For this review, take the finished solid that the model builds, in its own axes (mm). Face numbers are marked on the shaded views. A direction names the side the tool comes from. Give positions to 0.01 mm unless a question says otherwise; leave off trailing zeros. Order: outer loops, then holes, each group sorted by start corner. A loop starts at its lowest first (then second) coordinate and runs counter-clockwise, first axis right, second up.
Item 1: Machinability: for the marked faces 4, 5 and 6, which of the approach directions +Z, -Z, +X, -X, +Y, -Y give a long, thin tool a straight path to every point of the face, cutting with its end or side? Answer none if there is none.
Item 2: Consider section C-C (z = 0). Give the boundary of the cut face in (x, y).
Item 3: For probe 1 along Y at (x, z) = (-5.15, 0); probe 2 along Z at (x, y) = (-5.5, 13); probe 3 along Y at (x, z) = (-5.25, -0.5), list the stretches that pass through material, from the lowest coordinate up.
Item 4: Consider section A-A (x = -9). Give the boundary of the cut face in (y, z), plus the area to 3 significant figures.
Item 5: Consider section B-B (y = 10). Give the boundary of the cut face in (x, z), plus the area to 3 significant figures.
Item 6: The part is to be moulded in two halves that separate along Y. For the marked faces 1, 2 and 3, say which applies: released by +Y, released by -Y, zero draft, split by the parting line, or undercut.
Item 7: For P1, Ø1, axis at y = 9, z = 0.5, coming from the -X side; P2, Ø3, axis at y = 8.5, z = 4.5, coming from the -X side; P3, Ø1.5, axis at x = -3, y = 13, coming from the -Z side; P4, Ø2.5, axis at x = -8, y = 10, coming from the -Z side, all flat-tipped, find the tip position at first contact; note any pin that passes through.
Item 8: Consider section D-D (y = 15.25). Give the boundary of the cut face in (x, z).
```python
from build123d import *

# Parameters (mm, degrees)
BOSS_EXTRUDE1_DEPTH = 20
SKETCH2_R           = 2.1
CUT_EXTRUDE1_DEPTH  = 6


with BuildPart() as part:
    # Sketch1 → Boss-Extrude1 (new body)
    with BuildSketch(Plane(origin=(0, 0, 0), x_dir=(1, 0, 0), z_dir=(0, 1, 0))):
        with BuildLine():
            Line((-4.847127702, 5.487127702), (-4.847127702, 2.63))
            Line((-4.847127702, 2.63), (-9.847127702, 2.63))
            Line((-9.847127702, 2.63), (-9.847127702, -2.63))
            Line((-9.847127702, -2.63), (-4.847127702, -2.63))
            Line((-4.847127702, -2.63), (-4.847127702, -5.487127702))
            ThreePointArc((-4.847127702, -5.487127702), (-4.69775216, -5.84775216), (-4.337127702, -5.997127702))
            Line((-4.337127702, -5.997127702), (-3.607127702, -5.997127702))
            ThreePointArc((-3.607127702, -5.997127702), (-3.411959151, -5.958306263), (-3.246503243, -5.84775216))
            Line((-3.246503243, -5.84775216), (-0.149375542, -2.750624458))
            ThreePointArc((-0.149375542, -2.750624458), (-0.038821438, -2.585168551), (0, -2.39))
            Line((0, -2.39), (0, 2.39))
            ThreePointArc((0, 2.39), (-0.038821438, 2.585168551), (-0.149375542, 2.750624458))
            Line((-0.149375542, 2.750624458), (-3.246503243, 5.84775216))
            ThreePointArc((-3.246503243, 5.84775216), (-3.411959151, 5.958306263), (-3.607127702, 5.997127702))
            Line((-3.607127702, 5.997127702), (-4.337127702, 5.997127702))
            ThreePointArc((-4.337127702, 5.997127702), (-4.69775216, 5.84775216), (-4.847127702, 5.487127702))
        make_face()
    extrude(amount=BOSS_EXTRUDE1_DEPTH)

    # Sketch2 → Cut-Extrude1 (cut)
    with BuildSketch(Plane.ZY.offset(9.847127702)):
        with Locations((0, 10)):
            Circle(SKETCH2_R)
    extrude(amount=-CUT_EXTRUDE1_DEPTH, mode=Mode.SUBTRACT)


solid = part.part
```
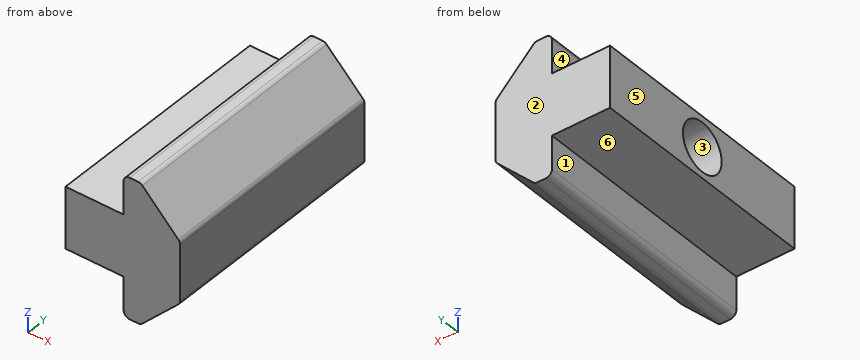
Resolved:
1. face 4: +Z, -X, +Y, -Y
1. face 5: +Z, -Z, -X, +Y, -Y
1. face 6: -Z, -X, +Y, -Y
2. outline: (-9.85, 0) - (0, 0) - (0, 20) - (-9.85, 20) - (-9.85, 12.1) - (-3.85, 12.1) - (-3.85, 7.9) - (-9.85, 7.9) - close
3. probe 1: y = 0 to 7.9, 12.1 to 20
3. probe 2: z = -2.63 to 2.63
3. probe 3: y = 0 to 7.96, 12.04 to 20
4. outline: (0, -2.63) - (20, -2.63) - (20, 2.63) - (0, 2.63) - close; hole circle Ø4.2 at (10, 0)
4. area: 91.3 mm2
5. outline: (-9.85, -2.63) - (-4.85, -2.63) - (-4.85, -5.49) arc R0.51 ccw to (-4.34, -6) - (-3.61, -6) arc R0.51 ccw to (-3.25, -5.85) - (-0.15, -2.75) arc R0.51 ccw to (0, -2.39) - (0, 2.39) arc R0.51 ccw to (-0.15, 2.75) - (-3.25, 5.85) arc R0.51 ccw to (-3.61, 6) - (-4.34, 6) arc R0.51 ccw to (-4.85, 5.49) - (-4.85, 2.63) - (-9.85, 2.63) - (-9.85, 2.1) - (-3.85, 2.1) - (-3.85, -2.1) - (-9.85, -2.1) - close
5. area: 47.6 mm2
6. face 1: zero draft
6. face 2: released by +Y
6. face 3: undercut
7. P1: stops at x = -3.85
7. P2: stops at x = -4.85
7. P3: stops at z = -6
7. P4: stops at z = -2.63
8. outline: (-9.85, -2.63) - (-4.85, -2.63) - (-4.85, -5.49) arc R0.51 ccw to (-4.34, -6) - (-3.61, -6) arc R0.51 ccw to (-3.25, -5.85) - (-0.15, -2.75) arc R0.51 ccw to (0, -2.39) - (0, 2.39) arc R0.51 ccw to (-0.15, 2.75) - (-3.25, 5.85) arc R0.51 ccw to (-3.61, 6) - (-4.34, 6) arc R0.51 ccw to (-4.85, 5.49) - (-4.85, 2.63) - (-9.85, 2.63) - close
